The listing builds one solid part. Answer for the finished solid, in the listing's coordinates (mm). Face numbers are marked on the shaded views. A direction names the side the tool comes from. Round coordinates to 2 decimals unless told otherwise and drop trailing zeros. Write each loop counter-clockwise with the first axis right and the second up, starting at its lowest first coordinate (ties: lowest second). Pieces come first, ordered by that corner, then holes.
(1) The mould has two halves that part along Z. Classify the marked faces 4, 5 and 6: +Z half, -Z half, draft (parallel to the pull), parting line (faces both ways), or undercut.
(2) Each of these flat-tipped pins is pushed along its axis until it touches: pin 1 Ø9.5 at (y, z) = (11.5, -37) entering from -X; pin 2 Ø1.6 at (x, z) = (-0.5, -59.5) entering from +Y; pin 3 Ø0.9 at (y, z) = (82.5, -96) entering from +X. Where does it stop, or does it pass through?
(3) A cutting plane is placed at C-C, the plane z = -38.5. Give the vertices of the cut face in (x, y).
(4) A cutting plane is placed at B-B, the plane x = -38. Give the vertices of the cut face in (y, z).
(5) For the marked faces 1, 2 and 3, determine the directions among +Z, -Z, +X, -X, +Y, -Y from which every point of the face is accessible in a straight line to the end or side of a thin tool.
(6) A cutting plane is placed at D-D, the plane y = 39. Give the vertices of the cut face in (x, z), and give its area (3 significant figures).
(7) A cutting plane is placed at A-A, the plane z = -113.5. Give the vertices of the cut face in (x, y), and give its area (3 significant figures).
(8) Find the intervals of material crossed by probe 1 along X at (y, z) = (17.5, -8); probe 2 along Y at (x, z) = (-61, -107), in increasing order.
Autodesk Inventor part; units mm, degrees
ref_plane "YZ Plane" through (0, 0, 0) normal (1, 0, 0) x (0, 1, 0)
ref_plane "XZ Plane" through (0, 0, 0) normal (0, 1, 0) x (-1, 0, 0)
ref_plane "XY Plane" through (0, 0, 0) normal (0, 0, 1) x (1, 0, 0)
sketch "Sketch1" plane through (0, 0, 0) normal (0, 1, 0) x (-1, 0, 0)
  line L0 (0, 0) -> (60, 0)
  line L1 (60, 0) -> (60, -60)
  line L2 (60, -60) -> (0, -60)
  line L3 (0, -60) -> (0, 0)
  dimension "d0" = 60
  dimension "d1" = 60
extrude "Extrusion1" add sketch "Sketch1" along normal blind 3
sketch "Sketch3" plane through (0, 3, 0) normal (0, 1, 0) x (1, 0, 0)
  line L0 (0, 60) -> (-60, 60)
  line L1 (0, 0) -> (0, 60)
  line L2 (-60, 60) -> (0, 60)
  line L3 (0, 60) -> (0, 58)
  line L4 (0, 58) -> (-60, 58)
  line L5 (-60, 58) -> (-60, 60)
  dimension "d4" = 2
extrude "Extrusion2" add sketch "Sketch3" along normal blind 18
sketch "Sketch4" plane through (0, 0, 0) normal (1, 0, 0) x (0, 0, -1)
  line L0 (0, 3) -> (58, 3)
  line L1 (0, 3) -> (0, 35)
  line L2 (60, 21) -> (58, 21)
  line L3 (0, 35) -> (58, 21)
  line L4 (58, 21) -> (58, 3)
  line L5 (58, 3) -> (0, 3)
  point P0 (0, 0)
  dimension "d7" = 32
extrude "Extrusion3" add sketch "Sketch4" against normal blind 2
sketch "Sketch5" plane through (-60, 0, -60) normal (-1, 0, 0) x (0, 0, 1)
  line L0 (2, 21) -> (0, 21)
  line L1 (0, 21) -> (2, 18)
  line L2 (2, 3) -> (2, 21)
  line L3 (2, 18) -> (2, 21)
  line L4 (2, 21) -> (0, 21)
  line L5 (0, 0) -> (0, 21)
  point P0 (60, 0)
  dimension "d10" = 3
extrude "Extrusion4" cut sketch "Sketch5" against normal blind 58
sketch "Sketch6" plane through (-60, 0, -60) normal (-1, 0, 0) x (0, 0, 1)
  line L0 (0, 0) -> (0, 21)
  line L1 (0, 21) -> (2, 21)
  line L2 (60, 35) -> (2, 21)
  line L3 (2, 21) -> (60, 35)
  line L4 (60, 35) -> (60, 0)
  line L5 (60, 0) -> (0, 0)
  line L6 (60, 0) -> (0, 0)
  line L7 (0, 0) -> (0, 21)
extrude "Extrusion5" add sketch "Sketch6" against normal blind 2
sketch "Sketch8" plane through (-58, 0, -60) normal (1, 0, 0) x (0, 0, -1)
  line L0 (-2, 3) -> (-60, 3)
  line L1 (-60, 3) -> (-58, 3)
  line L2 (-58, 3) -> (-58, 34.5172)
  line L3 (-2, 21) -> (-60, 35)
  line L4 (-58, 34.5172) -> (-60, 35)
  line L5 (-60, 35) -> (-60, 3)
  point P0 (-60, 0)
  dimension "d15" = 2
extrude "Extrusion6" add sketch "Sketch8" along normal blind 56
sketch "Sketch9" plane through (-60, 0, -60) normal (-1, 0, 0) x (0, 0, 1)
  line L0 (0, 21) -> (2, 21)
  line L1 (0, 21) -> (60, 21)
  line L2 (60, 21) -> (60, 81)
  line L3 (60, 81) -> (0, 81)
  line L4 (0, 81) -> (0, 21)
  point P0 (60, 0)
  dimension "d18" = 60
  dimension "d19" = 60
extrude "Extrusion7" add sketch "Sketch9" against normal blind 2
sketch "Sketch11" plane through (-58, 0, -60) normal (1, 0, 0) x (0, 0, -1)
  line L0 (0, 81) -> (-60, 81)
  line L1 (-60, 81) -> (66, 81)
  line L2 (66, 81) -> (66, 84)
  line L3 (66, 84) -> (-60, 84)
  line L4 (-60, 84) -> (-60, 81)
  point P0 (-60, 0)
  dimension "d26" = 3
  dimension "d27" = 126
extrude "Extrusion9" add sketch "Sketch11" against normal blind 13
sketch "Sketch12" plane through (-58, 84, 0) normal (0, 1, 0) x (1, 0, 0)
  circle A0 centre (-7, 119) radius 1
  line L0 (0, 126) -> (-13, 126)
  line L1 (0, 126) -> (0, 0)
  circle A1 centre (-7, 7) radius 1
  line L2 (0, 0) -> (-13, 0)
  point P0 (58, 0)
  dimension "d30" = 2
  dimension "d31" = 7
  dimension "d32" = 7
  dimension "d33" = 2
  dimension "d34" = 7
  dimension "d35" = 7
extrude "Extrusion10" cut sketch "Sketch12" against normal blind 13
sketch "Sketch13" plane through (-58, 84, 0) normal (0, 1, 0) x (1, 0, 0)
  circle A0 centre (-7, 7) radius 1
  line L0 (-8, 7) -> (-8, 119)
  line L1 (-8, 119) -> (-6, 119)
  line L2 (-6, 119) -> (-6, 7)
  line L3 (-6, 7) -> (-8, 7)
  circle A1 centre (-7, 119) radius 1
  point P0 (58, 0)
  dimension "d40" = 0
extrude "Extrusion11" cut sketch "Sketch13" against normal blind 10 contours A0 L0 A1 L2 | A1 L1 picked at (-6.9598, 118.6691)
sketch "Sketch14" plane through (-58, 84, 0) normal (0, 1, 0) x (1, 0, 0)
  point P0 (58, 0)
sketch "Sketch15" plane through (-58, 84, 0) normal (0, 1, 0) x (1, 0, 0)
  line L0 (-11.1798, 45.8772) -> (-2.4734, 45.8772)
  line L1 (-2.4734, 45.8772) -> (-2.4734, 82.1146)
  line L2 (-2.4734, 82.1146) -> (-11.1798, 82.1146)
  line L3 (-11.1798, 82.1146) -> (-11.1798, 45.8772)
  point P0 (58, 0)
extrude "Extrusion12" add sketch "Sketch15" against normal blind 3
properties part number "pickup_cup"
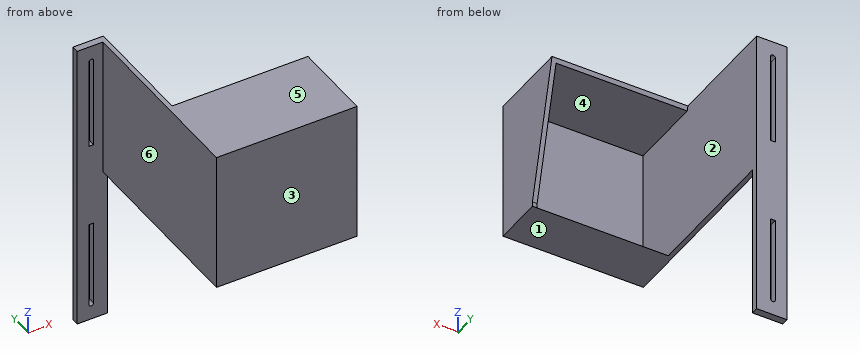
Solutions:
1. face 4: undercut
1. face 5: +Z half
1. face 6: draft
2. pin 1: stops at x = -60
2. pin 2: stops at y = 21
2. pin 3: stops at x = -58
3. outline: (-71, 81) - (-66, 81) - (-66, 84) - (-71, 84) - close; (-64, 81) - (-60, 81) - (-60, 0) - (0, 0) - (0, 25.71) - (-2, 25.71) - (-2, 3) - (-58, 3) - (-58, 84) - (-64, 84) - close
4. outline: (0, -60) - (21, -60) - (18, -58) - (3, -58) - (3, -2) - (34.52, -2) - (35, 0) - (0, 0) - close
5. face 1: -Z, +X, -X, -Y
5. face 2: +Y
5. face 3: +Z, -Z, +X, -X, -Y
6. outline: (-60, -60) - (-58, -60) - (-58, 0) - (-60, 0) - close
6. area: 120 mm2
7. outline: (-71, 81) - (-66, 81) - (-66, 84) - (-71, 84) - close; (-64, 81) - (-58, 81) - (-58, 84) - (-64, 84) - close
7. area: 33.0 mm2
8. probe 1: x = -60 to -58, -2 to 0
8. probe 2: y = 81 to 84
